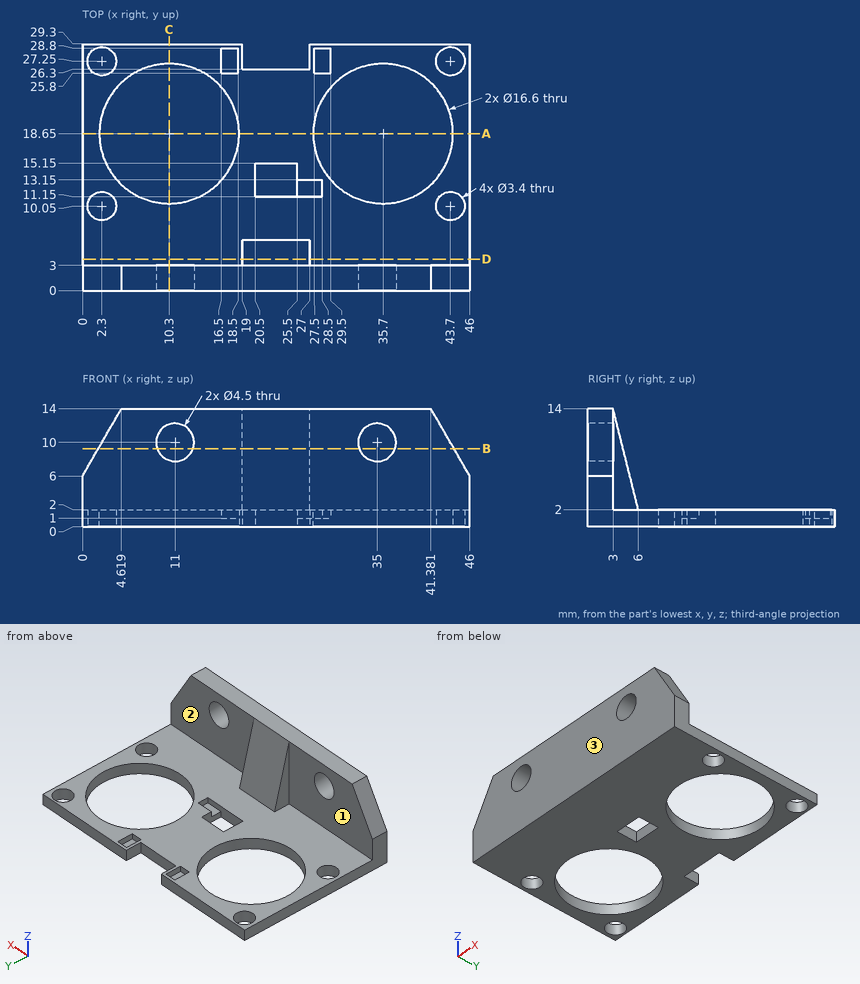
Geometry: see drawing. Coordinates: mm, zero at the bounding-box minimum. A direction names the side the tool comes from. Round coordinates to 2 decimals unless told otherwise and drop trailing zeros. Write each loop counter-clockwise with the first axis right and the second up, starting at its lowest first coordinate (ties: lowest second). Pieces come first, ordered by that corner, then holes. Notation, with made-up numbers: M -29.5,37 L 27.5,37 A34 ccw 27.5,74 Z; hole C 46,66 d10. An arc over 180 degrees is marked long. Answer in a Markdown table with one row per item. Add a question column.
(1) Reachability of the marked faces 1, 2 and 3 from +Z, -Z, +X, -X, +Y, -Y: full face, straight path, thin tool, end or side. Return the list, or none.
(2) Cut plane A-A, the plane y = 18.65. Return the cut outline in (x, z).
(3) Cut plane C-C, the plane x = 10.3. Return the cut outline in (y, z).
(4) Cut plane B-B, the plane z = 9.25. Return the cut outline in (x, y).
(5) Cut plane D-D, the plane y = 3.75. Return the cut outline in (x, z).
(6) Ray query, L1, parallel to Y at x = 32, z = 5; L2, parallel to Z at x = 40.5, y = 26.25; L3, parallel to X at y = 20.5, z = 0.75. Return the intervals inside material, ascending.
(7) Contact query for flat-ended pins moving along their axis: pin 1 (2 mm diameter, centred on x = 27, z = 8.5, fed in from +Y) (3 decimals); pin 2 (2 mm diameter, centred on x = 28, y = 28, fed in from +Z); pin 3 (3.5 mm diameter, centred on x = 33.5, z = 9.5, fed in from +Y). Output: stop coordinate, or through.
Established:
| question | item | result |
|---|---|---|
| 1 | face 1 | +Z, -X, +Y |
| 1 | face 2 | +Z, +X, +Y |
| 1 | face 3 | +Z, -Z, +X, -X, -Y |
| 2 | outline | M 0,0 L 2,0 L 2,2 L 0,2 Z; M 18.6,0 L 27.4,0 L 27.4,2 L 18.6,2 Z; M 44,0 L 46,0 L 46,2 L 44,2 Z |
| 3 | outline | M 0,0 L 10.35,0 L 10.35,2 L 3,2 L 3,7.86 L 0,7.86 Z; M 0,12.14 L 3,12.14 L 3,14 L 0,14 Z; M 26.95,0 L 29.3,0 L 29.3,2 L 26.95,2 Z |
| 4 | outline | M 1.88,0 L 8.88,0 L 8.88,3 L 1.88,3 Z; M 13.12,0 L 32.88,0 L 32.88,3 L 27,3 L 27,4.19 L 19,4.19 L 19,3 L 13.12,3 Z; M 37.12,0 L 44.12,0 L 44.12,3 L 37.12,3 Z |
| 5 | outline | M 0,0 L 46,0 L 46,2 L 27,2 L 27,11 L 19,11 L 19,2 L 0,2 Z |
| 6 | L1 | 0 to 3 |
| 6 | L2 | 0 to 2 |
| 6 | L3 | 0 to 2.21, 18.39 to 27.61, 43.79 to 46 |
| 7 | pin 1 | y = 4.625 |
| 7 | pin 2 | z = 2 |
| 7 | pin 3 | y = 3 |
